Source: CAD feature listing. Evaluate the final solid. Frame: model axes, mm. A direction names the side the tool comes from. Coordinates: 2 decimals unless noted, no trailing zeros. Order: outer loops, then holes, each group sorted by start corner. A loop starts at its lowest first (then second) coordinate and runs counter-clockwise, first axis right, second up. Notation, with made-up numbers: (25, 63.25) -> (63, 63.25) arc R22 ccw to (63, 99.25) -> close; hole circle Ø10 at (-0.5, -3). An arc over 180 degrees is marked (long way). Put each result on its own line as item: value.
from build123d import *

# Parameters (mm, degrees)
SKETCH1_W           = 300
SKETCH1_H           = 400
BOSS_EXTRUDE2_DEPTH = 117
SKETCH3_W           = 110
SKETCH3_H           = 110
CUT_EXTRUDE2_DEPTH  = 117
SKETCH5_W           = 270
SKETCH5_H           = 370
CUT_EXTRUDE3_DEPTH  = 102
SKETCH7_W           = 30
SKETCH7_H           = 15
CUT_EXTRUDE5_DEPTH  = 102
SKETCH8_W           = 10
SKETCH8_H           = 5
CUT_EXTRUDE7_DEPTH  = 90
SKETCH9_R           = 2.5
CUT_EXTRUDE8_DEPTH  = 90
SKETCH10_R          = 4
CUT_EXTRUDE9_DEPTH  = 90


with BuildPart() as part:
    # Sketch1 → Boss-Extrude2 (new body)
    with BuildSketch(Plane(origin=(0, 0, 0), x_dir=(1, 0, 0), z_dir=(0, 1, 0))):
        Rectangle(SKETCH1_W, SKETCH1_H)
    extrude(amount=BOSS_EXTRUDE2_DEPTH)

    # Sketch3 → Cut-Extrude2 (cut)
    with BuildSketch(Plane(origin=(0, 117, 0), x_dir=(1, 0, 0), z_dir=(0, 1, 0))):
        Rectangle(SKETCH3_W, SKETCH3_H)
    extrude(amount=-CUT_EXTRUDE2_DEPTH, mode=Mode.SUBTRACT)

    # Sketch5 → Cut-Extrude3 (cut)
    with BuildSketch(Plane(origin=(0, 117, 0), x_dir=(1, 0, 0), z_dir=(0, 1, 0))):
        Rectangle(SKETCH5_W, SKETCH5_H)
    extrude(amount=-CUT_EXTRUDE3_DEPTH, mode=Mode.SUBTRACT)

    # Sketch7 → Cut-Extrude5 (cut)
    with BuildSketch(Plane(origin=(0, 15, 0), x_dir=(1, 0, 0), z_dir=(0, 1, 0))):
        with Locations((0, 121.254101577)):
            Rectangle(SKETCH7_W, SKETCH7_H)
    extrude(amount=-CUT_EXTRUDE5_DEPTH, mode=Mode.SUBTRACT)

    # Sketch8 → Cut-Extrude7 (cut)
    with BuildSketch(Plane(origin=(150, 0, 0), x_dir=(0, 0, -1), z_dir=(1, 0, 0))):
        with Locations((-174.402323873, 69.081419449)):
            Rectangle(SKETCH8_W, SKETCH8_H)
    extrude(amount=-CUT_EXTRUDE7_DEPTH, mode=Mode.SUBTRACT)

    # Sketch9 → Cut-Extrude8 (cut)
    with BuildSketch(Plane.ZY.offset(150)):
        with Locations((181.740675273, 45.527316057)):
            Circle(SKETCH9_R)
        with Locations((165.218795702, 45.527316057)):
            Circle(SKETCH9_R)
        with Locations((144.15339925, 45.527316057)):
            Circle(SKETCH9_R)
        with Locations((123.088002798, 45.527316057)):
            Circle(SKETCH9_R)
    extrude(amount=-CUT_EXTRUDE8_DEPTH, mode=Mode.SUBTRACT)

    # Sketch10 → Cut-Extrude9 (cut)
    with BuildSketch(Plane(origin=(0, 15, 0), x_dir=(1, 0, 0), z_dir=(0, 1, 0))):
        with Locations((114.515150382, 165.914920232)):
            Circle(SKETCH10_R)
    extrude(amount=-CUT_EXTRUDE9_DEPTH, mode=Mode.SUBTRACT)


solid = part.part
1. Cut plane C-C on z = 37.5. Output: boundary loops of the cut face in (x, y), plus the area to 3 significant figures.
Numbers:
outline: (-150, 0) -> (-55, 0) -> (-55, 15) -> (-135, 15) -> (-135, 117) -> (-150, 117) -> close; (55, 0) -> (150, 0) -> (150, 117) -> (135, 117) -> (135, 15) -> (55, 15) -> close
area: 5,910 mm2
2. Cut plane A-A on x = -49. Output: boundary loops of the cut face in (y, z).
Numbers:
outline: (0, -200) -> (117, -200) -> (117, -185) -> (15, -185) -> (15, -55) -> (0, -55) -> close; (0, 55) -> (15, 55) -> (15, 185) -> (117, 185) -> (117, 200) -> (0, 200) -> close
3. Cut plane B-B on y = 53.5. Output: boundary loops of the cut face in (x, z), plus the area to 3 significant figures.
Numbers:
outline: (-150, -200) -> (150, -200) -> (150, 200) -> (-150, 200) -> close; hole (-135, -185) -> (135, -185) -> (135, 185) -> (-135, 185) -> close
area: 20,100 mm2
4. Set-up query: faces 1 (the flat face through (143, 71.581, 174)), 2 (the flat face through (15, 8, -121)), 3 (the flat face through (135, 67, 3)). Return all of +Z, -Z, +X, -X, +Y, -Y with unobstructed straight access to the full face (end or side cutting, diameter ignored); none if empty.
Numbers:
face 1: +X
face 2: +Y, -Y
face 3: +Y
5. Cut plane D-D on x = 4.5. Output: boundary loops of the cut face in (y, z).
Numbers:
outline: (0, -200) -> (117, -200) -> (117, -185) -> (15, -185) -> (15, -128.75) -> (0, -128.75) -> close; (0, -113.75) -> (15, -113.75) -> (15, -55) -> (0, -55) -> close; (0, 55) -> (15, 55) -> (15, 185) -> (117, 185) -> (117, 200) -> (0, 200) -> close
6. First-contact query: pin 1 (2 mm diameter, centred on x = -93.5, z = 31.5, fed in from +Y); pin 2 (3 mm diameter, centred on y = 45.53, z = 144.15, fed in from -X). Flat tips, straight axial feed; report the tip coordinate or a pass-through.
Numbers:
pin 1: stops at y = 15
pin 2: stops at x = 135
7. Ray query, line 1 along Z through (x, y) = (21, 51); line 2 along X through (y, z) = (42, -147); line 3 along Z through (x, y) = (-44.5, 14.5). Return the intervals inside material, ascending.
Numbers:
line 1: z = -200 to -185, 185 to 200
line 2: x = -150 to -135, 135 to 150
line 3: z = -200 to -55, 55 to 200
8. Pull-direction query (X, two-part tool) for faces 4 (the flat face through (-145, 117, -1)), 5 (the flat face through (55, 8, 1)), 6 (the flat face through (150, 58, 3)), 7 (the flat face through (-135, 67, 3)); classes: pulls with the +X half, pulls with the -X half, needs draft (parallel to the pull), parting line crosses it, or undercut.
Numbers:
face 4: needs draft
face 5: undercut
face 6: pulls with the +X half
face 7: undercut
